The listing builds one solid part. Answer for the finished solid, in the listing's coordinates (mm). Face numbers are marked on the shaded views. A direction names the side the tool comes from. Round coordinates to 2 decimals unless told otherwise and drop trailing zeros. Write each loop counter-clockwise with the first axis right and the second up, starting at its lowest first coordinate (ties: lowest second). Pieces come first, ordered by that corner, then holes.
(1) A cutting plane is placed at D-D, the plane y = 35. Give the vertices of the cut face in (x, z).
(2) Each of these flat-tipped pins is pushed along its axis until it touches: pin 1 Ø13 at (x, y) = (30.5, 36.5) entering from +Z; pin 2 Ø1.2 at (y, z) = (33.5, 6.5) entering from -X; pin 3 Ø3.5 at (x, z) = (40, 4.5) entering from -Y. Where does it stop, or does it pass through?
(3) A cutting plane is placed at C-C, the plane x = 34. Give the vertices of the cut face in (y, z), and give its area (3 significant figures).
(4) A cutting plane is placed at A-A, the plane y = 41.25. Give the vertices of the cut face in (x, z), and give its area (3 significant figures).
(5) A cutting plane is placed at B-B, the plane x = 0. Give the vertices of the cut face in (y, z).
(6) For the marked faces 4, 5, 6 and 7, determine the directions among +Z, -Z, +X, -X, +Y, -Y from which every point of the face is accessible in a straight line to the end or side of a thin tool.
(7) The mould has two halves that part along Y. Classify the marked faces 1, 2 and 3: +Y half, -Y half, draft (parallel to the pull), parting line (faces both ways), or undercut.
(8) Find the intervals of material crossed by probe 1 along Y at (x, z) = (32.3, 1.3); probe 2 along X at (y, z) = (41.5, 5); probe 3 along Y at (x, z) = (0, 1.6), in increasing order.
from build123d import *

# Parameters (mm, degrees)
SKETCH014_W     = 47.6
SKETCH014_H     = 24
SKETCH014_R     = 1.7
PAD003_DEPTH    = 10
POCKET011_DEPTH = 24.001
SKETCH016_R     = 2
POCKET012_DEPTH = 6
SKETCH017_W     = 7
SKETCH017_H     = 12
POCKET013_DEPTH = 6
SKETCH033_R     = 2
POCKET022_DEPTH = 5
SKETCH034_R     = 0.999503
POCKET023_DEPTH = 19.001
SKETCH020_W     = 18
SKETCH020_H     = 13
POCKET024_DEPTH = 7
SKETCH021_R     = 0.95
POCKET025_DEPTH = 5
POCKET026_DEPTH = 7
POCKET027_DEPTH = 8
POCKET028_DEPTH = 8
CHAMFER006_SIZE = 1
CHAMFER007_SIZE = 0.25


with BuildPart() as part:
    # Sketch014 → Pad003 (new body)
    with BuildSketch(Plane.XY):
        with Locations((20.7, 0)):
            Rectangle(SKETCH014_W, SKETCH014_H)
        Circle(SKETCH014_R, mode=Mode.SUBTRACT)
    extrude(amount=PAD003_DEPTH)

    # Sketch015 (on Face3 of Pad003) → Pocket011 (cut, through all)
    with BuildSketch(Plane.XZ.offset(12)):
        with BuildLine():
            Line((3, 10.1), (44.5, 10.1))
            Line((44.5, 4.5), (44.5, 10.1))
            ThreePointArc((44.5, 4.5), (43.181981, 7.68198), (40, 9))
            Line((40, 9), (10, 9))
            Line((10, 9), (10, 4))
            Line((10, 4), (3, 4))
            Line((3, 4), (3, 10.1))
        make_face()
    extrude(amount=-POCKET011_DEPTH, mode=Mode.SUBTRACT)

    # Sketch016 (on Face11 of Pocket011) → Pocket012 (cut)
    with BuildSketch(Plane.XZ.offset(12)):
        with Locations((40, 4.5)):
            Circle(SKETCH016_R)
    extrude(amount=-POCKET012_DEPTH, mode=Mode.SUBTRACT)

    # Sketch017 (on Face9 of Pocket012) → Pocket013 (cut)
    with BuildSketch(Plane.XY.offset(10)):
        Rectangle(SKETCH017_W, SKETCH017_H)
    extrude(amount=-POCKET013_DEPTH, mode=Mode.SUBTRACT)

    # Sketch033 (on Face1 of Pocket013) → Pocket022 (cut)
    with BuildSketch(Plane(origin=(0, 12, 0), x_dir=(-1, 0, 0), z_dir=(0, 1, 0))):
        with Locations((-40, 4.5)):
            Circle(SKETCH033_R)
    extrude(amount=-POCKET022_DEPTH, mode=Mode.SUBTRACT)

    # Sketch034 (on Face20 of Pocket022) → Pocket023 (cut, through all)
    with BuildSketch(Plane(origin=(0, 7, 0), x_dir=(-1, 0, 0), z_dir=(0, 1, 0))):
        with Locations((-40, 4.5)):
            Circle(SKETCH034_R)
    extrude(amount=-POCKET023_DEPTH, mode=Mode.SUBTRACT)

    # Sketch020 (on Face5 of Pocket013) → Pocket024 (cut)
    with BuildSketch(Plane.XY.offset(9)):
        with Locations((31.35, 2)):
            Rectangle(SKETCH020_W, SKETCH020_H)
    extrude(amount=-POCKET024_DEPTH, mode=Mode.SUBTRACT)

    # Sketch021 (on Face27 of Pocket024) → Pocket025 (cut)
    with BuildSketch(Plane.XY.offset(2)):
        with Locations((32.3, -1.2)):
            Circle(SKETCH021_R)
        with BuildLine():
            ThreePointArc((33.25, 5.4), (32.3, 6.35), (31.35, 5.4))
            Line((31.35, 5.4), (31.35, 5.2))
            ThreePointArc((31.35, 5.2), (32.3, 4.25), (33.25, 5.2))
            Line((33.25, 5.2), (33.25, 5.4))
        make_face()
    extrude(amount=-POCKET025_DEPTH, mode=Mode.SUBTRACT)

    # Sketch023 (on Face8 of Pocket025) → Pocket026 (cut)
    with BuildSketch(Plane.XY.offset(9)):
        Polygon((40.35, -4.5), (37.35, -4.5), (37.35, -7.5), (40.35, -5.98), align=None)
    extrude(amount=-POCKET026_DEPTH, mode=Mode.SUBTRACT)

    # Sketch024 (on Face12 of Pocket026) → Pocket027 (cut)
    with BuildSketch(Plane.XZ.offset(12)):
        with BuildLine():
            ThreePointArc((28.5, 2.3), (30.5, 4.3), (28.5, 6.3))
            Line((28.5, 6.3), (24.5, 6.3))
            ThreePointArc((24.5, 6.3), (22.5, 4.3), (24.5, 2.3))
            Line((24.5, 2.3), (28.5, 2.3))
        make_face()
    extrude(amount=-POCKET027_DEPTH, mode=Mode.SUBTRACT)

    # Sketch032 (on Face12 of Pocket027) → Pocket028 (cut)
    with BuildSketch(Plane.XZ.offset(12)):
        Polygon((31.392142, 10.286922), (27.849957, 3.99207), (30.144859, 3.99207), (33.687044, 10.286922), align=None)
    extrude(amount=-POCKET028_DEPTH, mode=Mode.SUBTRACT)

    # Chamfer006
    chamfer006_edges = [part.edges().sort_by_distance(p)[0] for p in [
        (-0.05, -12, 10),
        (-3.1, -9, 10),
        (-0.05, -6, 10),
        (3, -9, 10),
        (-0.05, 6, 10),
        (-3.1, 9, 10),
        (-0.05, 12, 10),
        (3, 9, 10),
        (10, 0, 9),
        (-3.1, -12, 5),
        (-3.1, 12, 5),
        (-3.1, 0, 0),
        (20.7, -12, 0),
        (20.7, 12, 0),
        (44.5, 0, 0),
    ]]
    chamfer(chamfer006_edges, length=CHAMFER006_SIZE)

    # Chamfer007
    chamfer007_edges = [part.edges().sort_by_distance(p)[0] for p in [
        (42, 12, 4.5),
        (38, -12, 4.5),
    ]]
    chamfer(chamfer007_edges, length=CHAMFER007_SIZE)


with BuildPart() as part_1:
    # Body002 placement: moved
    add(part.part.moved(Location((0, 31.9, 0))))


solid = part_1.part
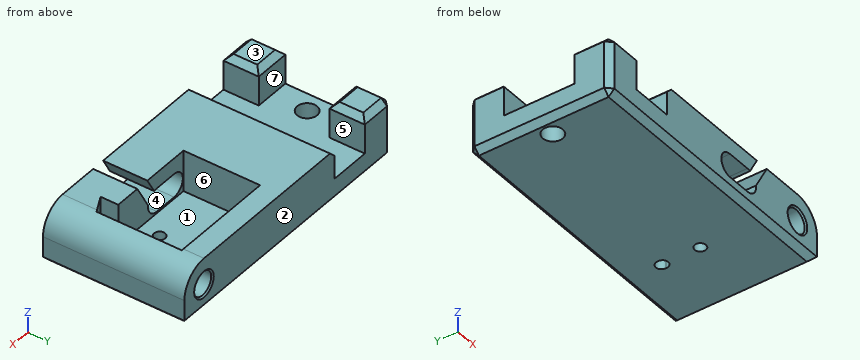
Solutions:
1. outline: (-3.1, 1) - (-2.1, 0) - (43.5, 0) - (44.5, 1) - (44.5, 4.5) arc R4.5 ccw to (40.35, 8.99) - (40.35, 5.44) arc R1 cw to (40.35, 3.56) - (40.35, 2) - (22.35, 2) - (22.35, 9) - (11, 9) - (10, 8) - (10, 4) - (-3.1, 4) - close
2. pin 1: stops at z = 9
2. pin 2: stops at x = 10
2. pin 3: stops at y = 25.9
3. outline: (19.9, 1) - (20.9, 0) - (42.9, 0) - (43.9, 1) - (43.9, 9) - (40.4, 9) - (40.4, 2) - (27.4, 2) - (27.4, 9) - (19.9, 9) - close
3. area: 124 mm2
4. outline: (-3.1, 1) - (-2.1, 0) - (43.5, 0) - (44.5, 1) - (44.5, 4.5) arc R4.5 ccw to (40, 9) - (11, 9) - (10, 8) - (10, 4) - (3, 4) - (3, 9) - (2, 10) - (-2.1, 10) - (-3.1, 9) - close; hole circle Ø4 at (40, 4.5)
4. area: 380 mm2
5. outline: (19.9, 1) - (20.9, 0) - (30.2, 0) - (30.2, 4) - (25.9, 4) - (25.9, 9) - (24.9, 10) - (20.9, 10) - (19.9, 9) - close; (33.6, 0) - (42.9, 0) - (43.9, 1) - (43.9, 9) - (42.9, 10) - (38.9, 10) - (37.9, 9) - (37.9, 4) - (33.6, 4) - close
6. face 4: -Y
6. face 5: +Z, +Y, -Y
6. face 6: +Z
6. face 7: +Z, -X
7. face 1: undercut
7. face 2: +Y half
7. face 3: draft
8. probe 1: y = 19.9 to 29.75, 31.65 to 36.15, 38.25 to 43.9
8. probe 2: x = -3.1 to 3, 10 to 38.06, 41.94 to 44.47
8. probe 3: y = 19.9 to 30.2, 33.6 to 43.9
